from build123d import *

# Parameters (mm, degrees)
ESQUISSE1_R        = 1.65
BOSS_EXTRU_1_DEPTH = 3
CHANFREIN1_SIZE    = 2


with BuildPart() as part:
    # Esquisse1 → Boss.-Extru.1 (new body)
    with BuildSketch(Plane.XY):
        with BuildLine():
            Line((-16, 0), (16, 0))
            ThreePointArc((16, 0), (18.121320344, 0.878679656), (19, 3))
            Line((19, 3), (19, 21.430548548))
            ThreePointArc((19, 21.430548548), (19.502411268, 25.885212805), (20.984403364, 30.11606971))
            Line((20.984403364, 30.11606971), (36.931973103, 63.194681617))
            ThreePointArc((36.931973103, 63.194681617), (0, 122), (-36.931973103, 63.194681617))
            Line((-36.931973103, 63.194681617), (-20.984403364, 30.11606971))
            ThreePointArc((-20.984403364, 30.11606971), (-19.502411268, 25.885212805), (-19, 21.430548548))
            Line((-19, 21.430548548), (-19, 3))
            ThreePointArc((-19, 3), (-18.121320344, 0.878679656), (-16, 0))
        make_face()
        with Locations((0, 116)):
            Circle(ESQUISSE1_R, mode=Mode.SUBTRACT)
        with Locations((19.780142429, 41.434276058)):
            Circle(ESQUISSE1_R, mode=Mode.SUBTRACT)
        with Locations((-19.780142429, 41.434276058)):
            Circle(ESQUISSE1_R, mode=Mode.SUBTRACT)
    extrude(amount=BOSS_EXTRU_1_DEPTH)

    # Chanfrein1
    chanfrein1_edges = [part.edges().sort_by_distance(p)[0] for p in [
        (-1.65, 116, 3),
        (18.130142429, 41.434276058, 3),
        (-21.430142429, 41.434276058, 3),
    ]]
    chamfer(chanfrein1_edges, length=CHANFREIN1_SIZE)


solid = part.part
Work out the finished part from the listing and answer in its coordinate system (mm). A direction names the side the tool comes from. Coordinates: 2 decimals unless noted, no trailing zeros. Order: outer loops, then holes, each group sorted by start corner. A loop starts at its lowest first (then second) coordinate and runs counter-clockwise, first axis right, second up. Notation, with made-up numbers: (-15.5, -5) - (-11.5, -5) arc R30 cw to (-11.5, 18) - close; hole circle Ø1 at (-23, 65). An arc over 180 degrees is marked (long way). Put each result on its own line as item: value. Start each with the question number.
1) For faces 1 (the flat face through (-19, 12, 1)), 2 (the flat face through (0, 0, 1)), determine the directions among +Z, -Z, +X, -X, +Y, -Y from which every point of the face is accessible in a straight line to the end or side of a thin tool.
2) For a pull along X with two mould halves and no side action, classify faces 3 (the cylindrical face through (20.54, 39.97, 0.49)), 4 (the flat face through (19, 12, 1)), 5 (the cylindrical face through (-19.517, 25.947, 1.479)), 6 (the cylindrical face through (1.159, 121.984, 1.479)) as released by +X, released by -X, zero draft, split by the parting line, or undercut.
3) Find section C-C (y = 116). Give the vertices of the cut face in (x, z), plus the area to 3 significant figures.
4) Find section A-A (x = 0). Give the vertices of the cut face in (y, z), plus the area to 3 significant figures.
5) Find section D-D (y = 72). Give the vertices of the cut face in (x, z), plus the area to 3 significant figures.
6) Find section B-B (z = 2.2). Give the vertices of the cut face in (x, y), plus the area to 3 significant figures.
7) Flat-ended cylindrical pins translate along their axes: pin 1 (1.5 mm diameter, centred on x = 29.5, z = 1.5, fed in from -Y); pin 2 (1 mm diameter, centred on x = -26.5, z = 0.5, fed in from -Y); pin 3 (2 mm diameter, centred on x = -19.78, y = 41.43, fed in from +Z). Find the tip coordinate at first contact, or state that the pin passes through.
8) Find the intervals of material crossed by line 1 (Y direction, x = 0, z = 0.3); line 2 (X direction, y = 14.5, z = 1.95); line 3 (Y direction, x = -1.5, z = 2.3), in increasing order. Write a range as from..to.
Results list:
1. face 1: +Z, -Z, -X, -Y
1. face 2: +Z, -Z, +X, -X, -Y
2. face 3: undercut
2. face 4: released by +X
2. face 5: released by -X
2. face 6: split by the parting line
3. outline: (-21.35, 0) - (-1.65, 0) - (-1.65, 1) - (-3.65, 3) - (-21.35, 3) - close; (1.65, 0) - (21.35, 0) - (21.35, 3) - (3.65, 3) - (1.65, 1) - close
3. area: 114 mm^2
4. outline: (0, 0) - (114.35, 0) - (114.35, 1) - (112.35, 3) - (0, 3) - close; (117.65, 0) - (122, 0) - (122, 3) - (119.65, 3) - (117.65, 1) - close
4. area: 352 mm^2
5. outline: (-40, 0) - (40, 0) - (40, 3) - (-40, 3) - close
5. area: 240 mm^2
6. outline: (-36.93, 63.19) - (-20.98, 30.12) arc R20 cw to (-19, 21.43) - (-19, 3) arc R3 ccw to (-16, 0) - (16, 0) arc R3 ccw to (19, 3) - (19, 21.43) arc R20 cw to (20.98, 30.12) - (36.93, 63.19) arc R41 ccw (long way) to start; hole circle Ø5.7 at (-19.78, 41.43); hole circle Ø5.7 at (0, 116); hole circle Ø5.7 at (19.78, 41.43)
6. area: 7,040 mm^2
7. pin 1: stops at y = 46.22
7. pin 2: stops at y = 40.52
7. pin 3: passes through
8. line 1: y = 0..114.35, 117.65..122
8. line 2: x = -19..19
8. line 3: y = 0..113.46, 118.54..121.97
